The model under review builds one solid part; all positions refer to its coordinate system, in mm. A direction names the side the tool comes from. Coordinates: 2 decimals unless noted, no trailing zeros. Use one line per item in the form item = value.
from build123d import *

# Parameters (mm, degrees)
SKETCH1_W           = 170
SKETCH1_H           = 250
BOSS_EXTRUDE1_DEPTH = 8
SKETCH2_W           = 5
SKETCH2_H           = 13
CUT_EXTRUDE1_DEPTH  = 8
SKETCH3_R           = 2
SKETCH3_W           = 6.8
SKETCH3_H           = 13
CUT_EXTRUDE2_DEPTH  = 8
FILLET1_R           = 8


with BuildPart() as part:
    # Sketch1 → Boss-Extrude1 (new body)
    with BuildSketch(Plane(origin=(0, 0, 0), x_dir=(1, 0, 0), z_dir=(0, 1, 0))):
        Rectangle(SKETCH1_W, SKETCH1_H)
    extrude(amount=BOSS_EXTRUDE1_DEPTH)

    # Sketch2 → Cut-Extrude1 (cut)
    with BuildSketch(Plane(origin=(0, 8, 0), x_dir=(1, 0, 0), z_dir=(0, 1, 0))):
        with Locations((82.5, 68.5)):
            Rectangle(SKETCH2_W, SKETCH2_H)
        with Locations((-82.5, 68.5)):
            Rectangle(SKETCH2_W, SKETCH2_H)
        with Locations((82.5, -68.5)):
            Rectangle(SKETCH2_W, SKETCH2_H)
        with Locations((-82.5, -68.5)):
            Rectangle(SKETCH2_W, SKETCH2_H)
    extrude(amount=-CUT_EXTRUDE1_DEPTH, mode=Mode.SUBTRACT)

    # Sketch3 → Cut-Extrude2 (cut)
    with BuildSketch(Plane(origin=(0, 8, 0), x_dir=(1, 0, 0), z_dir=(0, 1, 0))):
        with Locations(Location((-78, 118, 0), (0, 0, 270))):
            Circle(SKETCH3_R)
        with Locations(Location((78, 118, 0), (0, 0, 90))):
            Circle(SKETCH3_R)
        with Locations(Location((78, -118, 0), (0, 0, 270))):
            Circle(SKETCH3_R)
        with Locations(Location((-78, -118, 0), (0, 0, 90))):
            Circle(SKETCH3_R)
        with Locations(Location((-78, 0, 0), (0, 0, 270))):
            Circle(SKETCH3_R)
        with Locations(Location((78, 0, 0), (0, 0, 90))):
            Circle(SKETCH3_R)
        with Locations((-58.1, 68.5)):
            Rectangle(SKETCH3_W, SKETCH3_H)
        with Locations((58.1, 68.5)):
            Rectangle(SKETCH3_W, SKETCH3_H)
        with Locations((58.1, -68.5)):
            Rectangle(SKETCH3_W, SKETCH3_H)
        with Locations((-58.1, -68.5)):
            Rectangle(SKETCH3_W, SKETCH3_H)
    extrude(amount=-CUT_EXTRUDE2_DEPTH, mode=Mode.SUBTRACT)

    # Fillet1
    fillet1_edges = [part.edges().sort_by_distance(p)[0] for p in [
        (85, 4, 125),
        (-85, 4, 125),
        (-85, 4, -125),
        (85, 4, -125),
    ]]
    fillet(fillet1_edges, radius=FILLET1_R)


solid = part.part
Item 1: We need section A-A (y = 6). State how many separate pieces and enclosed holes the cut face has, plus the area to 3 significant figures.
Results found:
separate_pieces = 1
enclosed_holes = 10
area = 41,800 mm²
Item 2: To check wall thickness, follow L1, parallel to X at y = 5.75, z = 0; L2, parallel to X at y = 7, z = 68; L3, parallel to Z at x = -60.5, y = 4.75. State the ranges of each line that lie inside material, in increasing order. Write a range as from..to.
Results found:
L1 = -85..-80, -76..76, 80..85
L2 = -80..-61.5, -54.7..54.7, 61.5..80
L3 = -125..-75, -62..62, 75..125
Item 3: Clearance check with flat-ended pins moving along their axes: pin 1 (4 mm diameter, centred on x = 83, y = 5, fed in from -Z); pin 2 (1.5 mm diameter, centred on x = 82.5, y = 5.5, fed in from +Z); pin 3 (2.5 mm diameter, centred on x = -81.5, y = 4.5, fed in from -Z); pin 4 (2.5 mm diameter, centred on x = -78, z = 0, fed in from -Y). State where each tip first meets the part, or that it passes through.
Results found:
pin_1 = -123.93
pin_2 = 123.44
pin_3 = -124.31
pin_4 = through
Item 4: Draft analysis for pull direction Z (two halves, no side actions). For faces 6 (the face through (58, 4, 75)), 7 (the face through (85, 4, 1)), 8 (the face through (-1, 4, 125)), 9 (the face through (-82.719, 4.056, -122.594)), state which applies: released by +Z, released by -Z, zero draft, split by the parting line, or undercut.
Results found:
face_6 = undercut
face_7 = zero draft
face_8 = released by +Z
face_9 = released by -Z
Item 5: Tool access review of faces 1 (the face through (-58, 4, 62)), 2 (the face through (-82.719, 4.056, 122.594)), 3 (the face through (-80, 4, 69)), 4 (the face through (85, 4, 96)), 5 (the face through (80, 4, 69)): name each direction out of +Z, -Z, +X, -X, +Y, -Y from which nothing blocks a thin tool from reaching the whole face with its end or side.
Results found:
face_1 = +Y, -Y
face_2 = +Z, -X, +Y, -Y
face_3 = -X, +Y, -Y
face_4 = +Z, -Z, +X, +Y, -Y
face_5 = +X, +Y, -Y
